```python
from build123d import *

# Parameters (mm, degrees)
SKETCH1_W           = 110
SKETCH1_H           = 67
BOSS_EXTRUDE1_DEPTH = 3
CUT_EXTRUDE1_REACH  = 66.469
SKETCH2_W           = 24
SKETCH2_H           = 23
SKETCH2_W_2         = 17
SKETCH2_H_2         = 14
SKETCH2_W_3         = 15
SKETCH2_H_3         = 11
FILLET1_R           = 0.9


with BuildPart() as part:
    # Sketch1 → Boss-Extrude1 (new body)
    with BuildSketch(Plane.XY):
        Rectangle(SKETCH1_W, SKETCH1_H)
    extrude(amount=BOSS_EXTRUDE1_DEPTH)

    # Sketch2 → Cut-Extrude1 (cut, up to next)
    with BuildSketch(Plane.XY.offset(3), mode=Mode.PRIVATE) as cut_extrude1_sk1:
        with Locations((-31.75, 3.5)):
            Rectangle(SKETCH2_W, SKETCH2_H)
    cut_extrude1_tool1 = extrude(cut_extrude1_sk1.sketch, amount=-CUT_EXTRUDE1_REACH, mode=Mode.PRIVATE) & part.part
    # Sketch2 → Cut-Extrude1 (cut, up to next)
    with BuildSketch(Plane.XY.offset(3), mode=Mode.PRIVATE) as cut_extrude1_sk2:
        with Locations((0, 3.5)):
            Rectangle(SKETCH2_W_2, SKETCH2_H_2)
    cut_extrude1_tool2 = extrude(cut_extrude1_sk2.sketch, amount=-CUT_EXTRUDE1_REACH, mode=Mode.PRIVATE) & part.part
    # Sketch2 → Cut-Extrude1 (cut, up to next)
    with BuildSketch(Plane.XY.offset(3), mode=Mode.PRIVATE) as cut_extrude1_sk3:
        with Locations((31.75, 3.5)):
            Rectangle(SKETCH2_W, SKETCH2_H)
    cut_extrude1_tool3 = extrude(cut_extrude1_sk3.sketch, amount=-CUT_EXTRUDE1_REACH, mode=Mode.PRIVATE) & part.part
    # Sketch2 → Cut-Extrude1 (cut, up to next)
    with BuildSketch(Plane.XY.offset(3), mode=Mode.PRIVATE) as cut_extrude1_sk4:
        with Locations((44.5, 25)):
            Rectangle(SKETCH2_W_3, SKETCH2_H_3)
    cut_extrude1_tool4 = extrude(cut_extrude1_sk4.sketch, amount=-CUT_EXTRUDE1_REACH, mode=Mode.PRIVATE) & part.part
    add(cut_extrude1_tool1.solids().sort_by_distance((-31.75, 3.5, 3))[0], mode=Mode.SUBTRACT)
    add(cut_extrude1_tool2.solids().sort_by_distance((0, 3.5, 3))[0], mode=Mode.SUBTRACT)
    add(cut_extrude1_tool3.solids().sort_by_distance((31.75, 3.5, 3))[0], mode=Mode.SUBTRACT)
    add(cut_extrude1_tool4.solids().sort_by_distance((44.5, 25, 3))[0], mode=Mode.SUBTRACT)

    # Fillet1
    fillet1_edges = [part.edges().sort_by_distance(p)[0] for p in [
        (-55, 0, 3),
        (0, -33.5, 3),
        (-19.75, 3.5, 3),
        (-31.75, 15, 3),
        (-43.75, 3.5, 3),
        (-31.75, -8, 3),
        (8.5, 3.5, 3),
        (0, 10.5, 3),
        (-8.5, 3.5, 3),
        (0, -3.5, 3),
        (43.75, 3.5, 3),
        (31.75, 15, 3),
        (19.75, 3.5, 3),
        (31.75, -8, 3),
        (52, 25, 3),
        (44.5, 30.5, 3),
        (37, 25, 3),
        (44.5, 19.5, 3),
        (55, 0, 3),
        (0, 33.5, 3),
    ]]
    fillet(fillet1_edges, radius=FILLET1_R)


solid = part.part
```
Here's how the part is built. I have some questions about the finished solid (model axes, mm). A direction names the side the tool comes from. Coordinates: 2 decimals unless noted, no trailing zeros. Loops run counter-clockwise (first coordinate to the right, second up) from the corner with the lowest first, then second, coordinate; pieces in that order, holes last. Notation, with made-up numbers: (34, -3) - (56, -3) arc R13 ccw to (56, 1) - close; hole circle Ø11 at (-11.75, -29.75). An arc over 180 degrees is marked (long way). Answer as CSV lines item,"result".
Q1. If I drill on L1, parallel to X at y = -4.5, z = 0.7; L2, parallel to Y at x = 37.5, z = 1.8; L3, parallel to Y at x = 27, z = 1.45, over which ranges is the centre line in solid material (lowest first)? Write a range as [from, to].
Response:
L1,"[-55, -43.75], [-19.75, 19.75], [43.75, 55]"
L2,"[-33.5, -8], [15, 19.5], [30.5, 33.5]"
L3,"[-33.5, -8], [15, 33.5]"
Q2. If we section it at D-D, the plane y = 7: Write out the boundary of the cut face in (x, z).
Response:
outline,"(-55, 0) - (-43.75, 0) - (-43.75, 2.1) arc R0.9 ccw to (-44.65, 3) - (-54.1, 3) arc R0.9 ccw to (-55, 2.1) - close; (-19.75, 0) - (-8.5, 0) - (-8.5, 2.1) arc R0.9 ccw to (-9.4, 3) - (-18.85, 3) arc R0.9 ccw to (-19.75, 2.1) - close; (8.5, 0) - (19.75, 0) - (19.75, 2.1) arc R0.9 ccw to (18.85, 3) - (9.4, 3) arc R0.9 ccw to (8.5, 2.1) - close; (43.75, 0) - (55, 0) - (55, 2.1) arc R0.9 ccw to (54.1, 3) - (44.65, 3) arc R0.9 ccw to (43.75, 2.1) - close"
Q3. For faces 5 (the face through (-1, -7, 3)), 6 (the face through (32, -8, 1)), which set-ups out of +Z, -Z, +X, -X, +Y, -Y let a thin tool reach every point of the face, with its end or its side?
Response:
face 5,"+Z, +X, -X, +Y, -Y"
face 6,"+Z, -Z"
Q4. We'd pull the mould along X, two halves only. Please class faces 1 (the face through (43.75, 3, 1)), 2 (the face through (-1, 33.5, 1)), 3 (the face through (44, 19.5, 1)), 4 (the face through (-55, 0, 1)): pulls with the +X half, pulls with the -X half, needs draft (parallel to the pull), parting line crosses it, or undercut.
Response:
face 1,"undercut"
face 2,"needs draft"
face 3,"undercut"
face 4,"pulls with the -X half"
Q5. If we section it at B-B, the plane y = 28: Write out the boundary of the cut face in (x, z), and give its area (3 significant figures).
Response:
outline,"(-55, 0) - (37, 0) - (37, 2.1) arc R0.9 ccw to (36.1, 3) - (-54.1, 3) arc R0.9 ccw to (-55, 2.1) - close; (52, 0) - (55, 0) - (55, 2.1) arc R0.9 ccw to (54.1, 3) - (52.9, 3) arc R0.9 ccw to (52, 2.1) - close"
area,"284 mm2"
Q6. If we section it at C-C, the plane z = 0.85: Write out the boundary of the cut face in (x, y), and give its area (3 significant figures).
Response:
outline,"(-55, -33.5) - (55, -33.5) - (55, 33.5) - (-55, 33.5) - close; hole (-43.75, -8) - (-19.75, -8) - (-19.75, 15) - (-43.75, 15) - close; hole (-8.5, -3.5) - (8.5, -3.5) - (8.5, 10.5) - (-8.5, 10.5) - close; hole (19.75, -8) - (43.75, -8) - (43.75, 15) - (19.75, 15) - close; hole (37, 19.5) - (52, 19.5) - (52, 30.5) - (37, 30.5) - close"
area,"5,860 mm2"
Q7. If we section it at A-A, the plane x = -26.5: Write out the boundary of the cut face in (y, z).
Response:
outline,"(-33.5, 0) - (-8, 0) - (-8, 2.1) arc R0.9 ccw to (-8.9, 3) - (-32.6, 3) arc R0.9 ccw to (-33.5, 2.1) - close; (15, 0) - (33.5, 0) - (33.5, 2.1) arc R0.9 ccw to (32.6, 3) - (15.9, 3) arc R0.9 ccw to (15, 2.1) - close"
